from build123d import *

# Parameters (mm, degrees)
SKETCH1_R      = 1.45
MID_BODY_DEPTH = 2.3
SKETCH2_R      = 2
TOP_HEAD_DEPTH = 1


with BuildPart() as part:
    # Sketch1 → MID BODY (new, symmetric)
    with BuildSketch(Plane(origin=(0, 0, 0), x_dir=(1, 0, 0), z_dir=(0, 1, 0))):
        with Locations(Location((0, 0, 0), (0, 0, 270))):
            Circle(SKETCH1_R)
    extrude(amount=MID_BODY_DEPTH, both=True)

    # Sketch2 → TOP HEAD (add)
    with BuildSketch(Plane(origin=(0, 2.3, 0), x_dir=(1, 0, 0), z_dir=(0, 1, 0))):
        with Locations(Location((0, 0, 0), (0, 0, 270))):
            Circle(SKETCH2_R)
    top_head = extrude(amount=TOP_HEAD_DEPTH)

    # BOTTOM HEAD: TOP HEAD across plane
    add(top_head.mirror(Plane.ZX))


solid = part.part
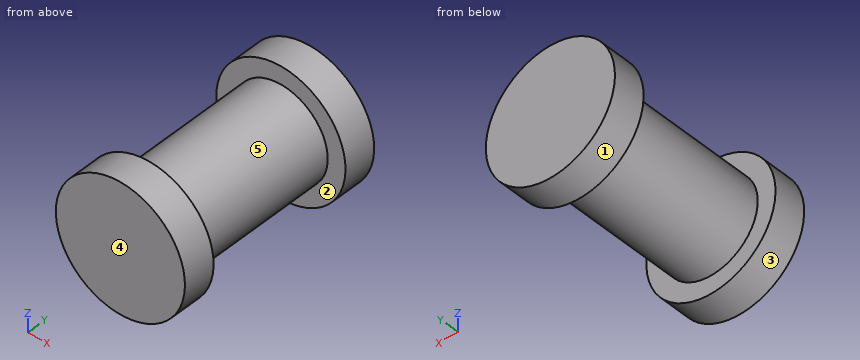
For this review, take the finished solid that the model builds, in its own axes (mm). Face numbers are marked on the shaded views. A direction names the side the tool comes from. Give positions to 0.01 mm unless a question says otherwise; leave off trailing zeros. Loops run counter-clockwise (first coordinate to the right, second up) from the corner with the lowest first, then second, coordinate; pieces in that order, holes last. Notation, with made-up numbers: M -17.5,39 L 15.5,39 A33 cw 15.5,69 Z; hole C -14.5,-39.75 d10. An arc over 180 degrees is marked long. Put each result on its own line as item: value. Start each with the question number.
(1) The part is to be moulded in two halves that separate along Y. For the marked faces 3, 4 and 5, say which applies: +Y half, -Y half, draft (parallel to the pull), parting line (faces both ways), or undercut.
(2) Wall thickness on L1, parallel to Y at x = 1.85, z = 0; L2, parallel to Z at x = 0.4, y = 3; L3, parallel to Z at x = -1.5, y = -2.5: over which ranges is each line inside the solid? List them lowest first.
(3) Add section A-A, the plane z = 1.6. Write out the cut boundary in (x, y).
(4) For pin 1 (1.5 mm diameter, centred on x = 1.5, y = 2, fed in from -Z); pin 2 (2 mm diameter, centred on y = -1, z = -1, fed in from -X), all flat-tipped, find the tip position at first contact; note any pin that passes through.
(5) Add section C-C, the plane z = 0. Write out the cut boundary in (x, y), then the cut area to 3 significant figures.
(6) Add section D-D, the plane y = 0.5. Write out the cut boundary in (x, z), then the cut area to 3 significant figures.
(7) Machinability: for the marked faces 1 and 2, which of the approach directions +Z, -Z, +X, -X, +Y, -Y give a long, thin tool a straight path to every point of the face, cutting with its end or side? Answer none if there is none.
(8) Add section B-B, the plane x = 0. Write out the cut boundary in (y, z).
Result:
1. face 3: draft
1. face 4: -Y half
1. face 5: undercut
2. L1: y = -3.3 to -2.3, 2.3 to 3.3
2. L2: z = -1.96 to 1.96
2. L3: z = -1.32 to 1.32
3. outline: M -1.2,-3.3 L 1.2,-3.3 L 1.2,-2.3 L -1.2,-2.3 Z; M -1.2,2.3 L 1.2,2.3 L 1.2,3.3 L -1.2,3.3 Z
4. pin 1: stops at z = -1.83
4. pin 2: stops at x = -1.45
5. outline: M -2,-3.3 L 2,-3.3 L 2,-2.3 L 1.45,-2.3 L 1.45,2.3 L 2,2.3 L 2,3.3 L -2,3.3 L -2,2.3 L -1.45,2.3 L -1.45,-2.3 L -2,-2.3 Z
5. area: 21.3 mm^2
6. outline: C 0,0 d2.9
6. area: 6.61 mm^2
7. face 1: +Y, -Y
7. face 2: none
8. outline: M -3.3,-2 L -2.3,-2 L -2.3,-1.45 L 2.3,-1.45 L 2.3,-2 L 3.3,-2 L 3.3,2 L 2.3,2 L 2.3,1.45 L -2.3,1.45 L -2.3,2 L -3.3,2 Z
